```python
from build123d import *

# Parameters (mm, degrees)
SKETCH001_R   = 1.65
EXTRUDE_DEPTH = 40
PAD_DEPTH     = 27


with BuildPart() as extrude_body:
    # Sketch001 → Extrude (new body, symmetric)
    with BuildSketch(Plane.XZ):
        with BuildLine():
            ThreePointArc((20, 0), (27.266003, 5.641182), (23.601647, 14.078612))
            Line((0, 27), (23.601647, 14.078612))
            Line((0, 0), (0, 27))
            Line((0, 0), (20, 0))
        make_face()
        with Locations((20, 7.5)):
            Circle(SKETCH001_R, mode=Mode.SUBTRACT)
    extrude(amount=EXTRUDE_DEPTH, both=True)


with BuildPart() as common:
    # Sketch → Pad (new body)
    with BuildSketch(Plane.XY):
        Polygon((0, 22.1), (4, 22.1), (4, 6.1), (27.5, 6.1), (27.5, 2.1), (8, 2.1), (8, -2.1), (27.5, -2.1), (27.5, -6.1), (0, -6.1), (0, -2.1), (4, -2.1), (4, 2.1), (0, 2.1), align=None)
    extrude(amount=PAD_DEPTH)

    # Common: intersect Extrude body
    add(extrude_body.part, mode=Mode.INTERSECT)


solid = common.part
```
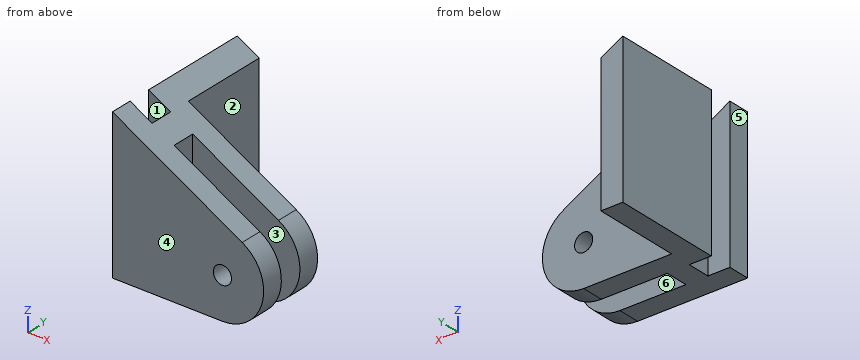
Work out the finished part from the listing and answer in its coordinate system (mm). Face numbers are marked on the shaded views. A direction names the side the tool comes from. Coordinates: 2 decimals unless noted, no trailing zeros. Loops run counter-clockwise (first coordinate to the right, second up) from the corner with the lowest first, then second, coordinate; pieces in that order, holes last.
1) For a pull along Y with two mould halves and no side action, classify the marked faces 4, 5 and 6 as +Y half, -Y half, draft (parallel to the pull), parting line (faces both ways), or undercut.
Results:
face 4: -Y half
face 5: draft
face 6: undercut
2) Consider probe 1 along X at (y, z) = (3.6, 7.5); probe 2 along Y at (x, z) = (16.25, 1.75); probe 3 along X at (y, z) = (19, 22.25). Determine where each line is inside the solid, lowest interval first.
Results:
probe 1: x = 0 to 18.35, 21.65 to 27.5
probe 2: y = -6.1 to -2.1, 2.1 to 6.1
probe 3: x = 0 to 4
3) For the marked faces 1, 2 and 3, determine the directions among +Z, -Z, +X, -X, +Y, -Y from which every point of the face is accessible in a straight line to the end or side of a thin tool.
Results:
face 1: +Z, -Z, -X
face 2: +Z, -Z, +X, +Y
face 3: +Z, -Z, +X
4) Section A-A (z = 7.5) is taken. Give the vertices of the cut face in (x, y).
Results:
outline: (0, -6.1) - (18.35, -6.1) - (18.35, -2.1) - (8, -2.1) - (8, 2.1) - (18.35, 2.1) - (18.35, 6.1) - (4, 6.1) - (4, 22.1) - (0, 22.1) - (0, 2.1) - (4, 2.1) - (4, -2.1) - (0, -2.1) - close; (21.65, -6.1) - (27.5, -6.1) - (27.5, -2.1) - (21.65, -2.1) - close; (21.65, 2.1) - (27.5, 2.1) - (27.5, 6.1) - (21.65, 6.1) - close
5) Flat-ended cylindrical pins translate along their axes: pin 1 (1.5 mm diameter, centred on x = 14.5, z = 3, fed in from +Y); pin 2 (3 mm diameter, centred on y = 0.5, z = 10.5, fed in from -X); pin 3 (2 mm diameter, centred on y = 1, z = 13.5, fed in from +X). Find the tip coordinate at first contact, or state that the pin passes through.
Results:
pin 1: stops at y = 6.1
pin 2: stops at x = 4
pin 3: stops at x = 8
6) Section B-B (x = 12.25) is taken. Give the vertices of the cut face in (y, z).
Results:
outline: (-6.1, 0) - (-2.1, 0) - (-2.1, 20.29) - (-6.1, 20.29) - close; (2.1, 0) - (6.1, 0) - (6.1, 20.29) - (2.1, 20.29) - close
7) Section D-D (z = 12) is taken. Give the vertices of the cut face in (x, y), plus the area to 3 significant figures.
Results:
outline: (0, -6.1) - (26, -6.1) - (26, -2.1) - (8, -2.1) - (8, 2.1) - (26, 2.1) - (26, 6.1) - (4, 6.1) - (4, 22.1) - (0, 22.1) - (0, 2.1) - (4, 2.1) - (4, -2.1) - (0, -2.1) - close
area: 289 mm2
8) Section C-C (y = 5.5) is taken. Give the vertices of the cut face in (x, z).
Results:
outline: (0, 0) - (20, 0) arc R7.5 ccw to (23.6, 14.08) - (0, 27) - close; hole circle Ø3.3 at (20, 7.5)
